Verification items for the finished model (mm, model axes). Face numbers are marked on the shaded views. A direction names the side the tool comes from. Coordinates: 2 decimals unless noted, no trailing zeros. Order: outer loops, then holes, each group sorted by start corner. A loop starts at its lowest first (then second) coordinate and runs counter-clockwise, first axis right, second up. Notation, with made-up numbers: (4.5, -5.75) -> (57.5, -5.75) arc R22 cw to (57.5, 22.25) -> close; hole circle Ø7 at (-8, 4). An arc over 180 degrees is marked (long way). Use CSV: the item, a comma, the result in double quotes. Start each with the question number.
1) Sectioned sample at C-C on y = 0. Record the boundary of the cut face in (x, z) (3 decimals), then the cut area to 3 significant figures.
2) Sectioned sample at B-B on z = -15.25. Record the boundary of the cut face in (x, y), then the cut area to 3 significant figures.
3) Sectioned sample at A-A on x = 0. Give the number of separate pieces and of enclosed holes in the cut face, then the cut area to 3 significant figures.
4) Go/stop test with flat-tipped pins: pin 1 (0.5 mm diameter, centred on y = 4.5, z = -15, fed in from -X); pin 2 (1.5 mm diameter, centred on y = -4, z = -11, fed in from +X); pin 3 (2 mm diameter, centred on x = 0, z = -16.5, fed in from +Y). Record where each tip stops, or that it passes through.
5) Scan lines: line 1 along Z through (x, y) = (1.25, -1.5); line 2 along Z through (x, y) = (-1.5, 4.25); line 3 along Y through (x, z) = (-4, -1). Record each from-to range of solid material in increasing order.
6) Sectioned sample at D-D on z = -6.75. Record the boundary of the cut face in (x, y), then the cut area to 3 significant figures.
7) Release check for a two-part mould opening along X. For the marked faces 5 and 6 record: released by +X, released by -X, zero draft, split by the parting line, or undercut.
8) Tool access check on the marked faces 1, 2, 3 and 4. Record the directions out of +Z, -Z, +X, -X, +Y, -Y that give a thin tool (end or side, any length) a straight path to the whole face; none if there is none.
from build123d import *

# Parameters (mm, degrees)
SKETCH1_R           = 6
BOSS_EXTRUDE1_DEPTH = 14
SKETCH2_R           = 6.925
BOSS_EXTRUDE2_DEPTH = 1.6
CHAMFER1_SIZE       = 1.4
SKETCH3_R           = 4.45
BOSS_EXTRUDE3_DEPTH = 1.2
FILLET1_R           = 1.15
SKETCH5_W           = 2
SKETCH5_H           = 0.47
BOSS_EXTRUDE4_DEPTH = 3.3
SKETCH6_R           = 0.395429062
CUT_EXTRUDE1_DEPTH  = 22.84242775


with BuildPart() as part:
    # Sketch1 → Boss-Extrude1 (new body)
    with BuildSketch(Plane.XY):
        Circle(SKETCH1_R)
    extrude(amount=-BOSS_EXTRUDE1_DEPTH)

    # Sketch2 → Boss-Extrude2 (add)
    with BuildSketch(Plane.XY):
        Circle(SKETCH2_R)
    extrude(amount=BOSS_EXTRUDE2_DEPTH)

    # Chamfer1
    chamfer1_edges = [part.edges().sort_by_distance(p)[0] for p in [
        (-6.925, 0, 1.6),
    ]]
    chamfer(chamfer1_edges, length=CHAMFER1_SIZE)

    # Sketch3 → Boss-Extrude3 (add)
    with BuildSketch(Plane.XY.offset(1.6)):
        Circle(SKETCH3_R)
    extrude(amount=BOSS_EXTRUDE3_DEPTH)

    # Fillet1
    fillet1_edges = [part.edges().sort_by_distance(p)[0] for p in [
        (-6, 0, -14),
    ]]
    fillet(fillet1_edges, radius=FILLET1_R)

    # Sketch5 → Boss-Extrude4 (add)
    with BuildSketch(Plane(origin=(0, 0, -14), x_dir=(-1, 0, 0), z_dir=(0, 0, -1))):
        with Locations((0, -4.235)):
            Rectangle(SKETCH5_W, SKETCH5_H)
        with Locations((0, 4.235)):
            Rectangle(SKETCH5_W, SKETCH5_H)
    extrude(amount=BOSS_EXTRUDE4_DEPTH)

    # Sketch6 → Cut-Extrude1 (cut, through all)
    with BuildSketch(Plane(origin=(0, 4.47, 0), x_dir=(1, 0, 0), z_dir=(0, 1, 0))):
        with Locations(Location((0, 16.408005075, 0), (0, 0, 270))):
            Circle(SKETCH6_R)
    extrude(amount=-CUT_EXTRUDE1_DEPTH, mode=Mode.SUBTRACT)


solid = part.part
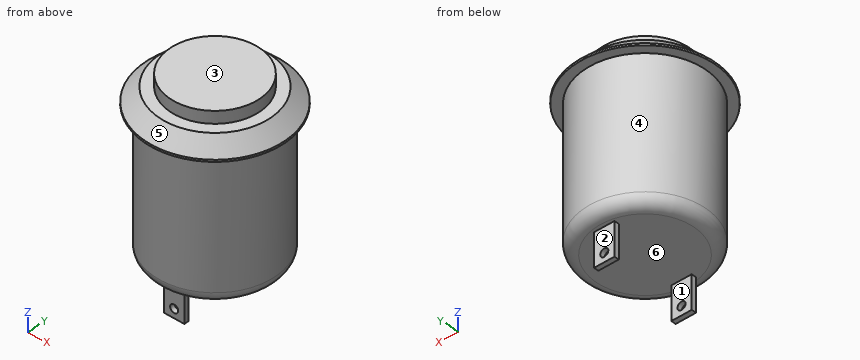
Answers follow:
1,outline,"(-6.925, 0) -> (-6, 0) -> (-6, -12.85) arc R1.15 ccw to (-4.85, -14) -> (4.85, -14) arc R1.15 ccw to (6, -12.85) -> (6, 0) -> (6.925, 0) -> (6.925, 0.2) -> (5.525, 1.6) -> (4.45, 1.6) -> (4.45, 2.8) -> (-4.45, 2.8) -> (-4.45, 1.6) -> (-5.525, 1.6) -> (-6.925, 0.2) -> close"
1,area,"198 mm²"
2,outline,"(-1, -4.47) -> (1, -4.47) -> (1, -4) -> (-1, -4) -> close; (-1, 4) -> (1, 4) -> (1, 4.47) -> (-1, 4.47) -> close"
2,area,"1.88 mm²"
3,separate pieces,"3"
3,enclosed holes,"0"
3,area,"201 mm²"
4,pin 1,"stops at x = -1"
4,pin 2,"stops at x = 5.04"
4,pin 3,"stops at y = 4.47"
5,line 1,"z = -14 to 2.8"
5,line 2,"z = -14 to 1.6"
5,line 3,"y = -4.47 to 4.47"
6,outline,"circle Ø12 at (0, 0)"
6,area,"113 mm²"
7,face 5,"split by the parting line"
7,face 6,"zero draft"
8,face 1,"-Z, +X, -X"
8,face 2,"-Z, +X, -X, +Y"
8,face 3,"+Z, +X, -X, +Y, -Y"
8,face 4,"-Z"
